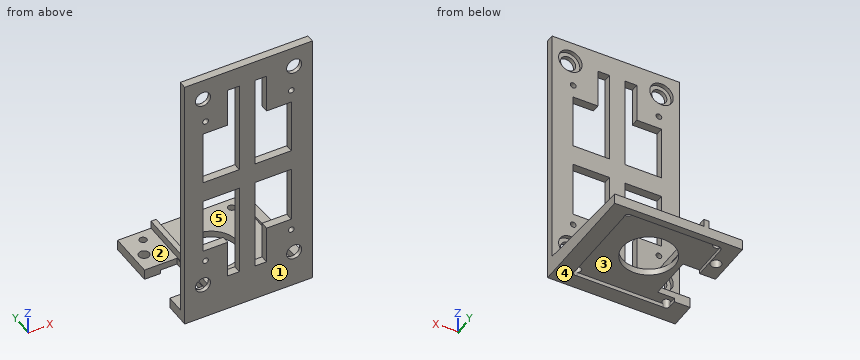
from build123d import *

# Parameters (mm, degrees)
SKETCH_1_R           = 2.9
SKETCH_1_R_2         = 1.1
EXTRUDE_1_DEPTH      = 3
SKETCH_2_R           = 4.5
CUT_EXTRUDE_1_DEPTH  = 1.5
SKETCH_3_W           = 49
SKETCH_3_H           = 4
EXTRUDE_2_DEPTH      = 42
EXTRUDE_2_DEPTH_BACK = 3
SKETCH_4_R           = 1.4
SKETCH_4_W           = 14.760499622
SKETCH_4_H           = 17
SKETCH_4_R_2         = 10
SKETCH_4_R_3         = 2
CUT_EXTRUDE_2_DEPTH  = 5
SKETCH_5_R           = 10
CUT_EXTRUDE_3_DEPTH  = 1.5
EXTRUDE_4_DEPTH      = 3.5
SKETCH_9_W           = 2
SKETCH_9_H           = 3
EXTRUDE_5_DEPTH      = 42
SKETCH_10_W          = 3
SKETCH_10_H          = 5.066593596
EXTRUDE_6_DEPTH      = 21


with BuildPart() as part:
    # 草图1 → 凸台-拉伸1 (new body)
    with BuildSketch(Plane(origin=(0, 0, 0), x_dir=(1, 0, 0), z_dir=(0, 1, 0))):
        Polygon((-42, 46), (-42, -1), (-42, -48), (0, -48), (7, -48), (7, 47), (7, 50), (-42, 50), align=None)
        with Locations((-35, -40)):
            Circle(SKETCH_1_R, mode=Mode.SUBTRACT)
        with Locations((-34, -30)):
            Circle(SKETCH_1_R_2, mode=Mode.SUBTRACT)
        Polygon((-35, -25), (-35, -4), (-21.05, -4), (-21.05, -40), (-25.5, -40), (-25.5, -25), align=None, mode=Mode.SUBTRACT)
        with Locations((0, -40)):
            Circle(SKETCH_1_R, mode=Mode.SUBTRACT)
        with Locations((-1.1, -30)):
            Circle(SKETCH_1_R_2, mode=Mode.SUBTRACT)
        Polygon((-1.1, -4), (-1.1, -25), (-10.6, -25), (-10.6, -40), (-15.05, -40), (-15.05, -4), align=None, mode=Mode.SUBTRACT)
        Polygon((-21.05, 4), (-35, 4), (-35, 25.5), (-25.5, 25.5), (-25.5, 40), (-21.05, 40), align=None, mode=Mode.SUBTRACT)
        with Locations((-34, 30)):
            Circle(SKETCH_1_R_2, mode=Mode.SUBTRACT)
        with Locations((-35, 40)):
            Circle(SKETCH_1_R, mode=Mode.SUBTRACT)
        Polygon((-10.6, 25.5), (-1.1, 25.5), (-1.1, 4), (-15.05, 4), (-15.05, 40), (-10.6, 40), align=None, mode=Mode.SUBTRACT)
        with Locations((-1.1, 30)):
            Circle(SKETCH_1_R_2, mode=Mode.SUBTRACT)
        with Locations((0, 40)):
            Circle(SKETCH_1_R, mode=Mode.SUBTRACT)
    extrude(amount=EXTRUDE_1_DEPTH)

    # 草图2 → 切除-拉伸1 (cut)
    with BuildSketch(Plane(origin=(0, 3, 0), x_dir=(1, 0, 0), z_dir=(0, 1, 0))):
        with Locations((-35, 40)):
            Circle(SKETCH_2_R)
        with Locations((0, 40)):
            Circle(SKETCH_2_R)
        with Locations((0, -40)):
            Circle(SKETCH_2_R)
        with Locations((-35, -40)):
            Circle(SKETCH_2_R)
    extrude(amount=-CUT_EXTRUDE_1_DEPTH, mode=Mode.SUBTRACT)

    # 草图3 → 凸台-拉伸2 (add, two sides)
    with BuildSketch(Plane(origin=(0, 3, 0), x_dir=(1, 0, 0), z_dir=(0, 1, 0))) as extrude_2_sk:
        with Locations((-17.5, 52)):
            Rectangle(SKETCH_3_W, SKETCH_3_H)
    extrude(amount=EXTRUDE_2_DEPTH)
    extrude(extrude_2_sk.sketch, amount=-EXTRUDE_2_DEPTH_BACK)

    # 草图4 → 切除-拉伸2 (cut, through all)
    with BuildSketch(Plane.XY.offset(-50)):
        with Locations((-34.5, 7)):
            Circle(SKETCH_4_R)
        with Locations((-36.880249811, 18.5)):
            Rectangle(SKETCH_4_W, SKETCH_4_H)
        with Locations((-34.5, 41)):
            Circle(SKETCH_4_R)
        with Locations((-0.5, 41)):
            Circle(SKETCH_4_R)
        with Locations((-0.5, 7)):
            Circle(SKETCH_4_R)
        with Locations((-17.5, 25)):
            Circle(SKETCH_4_R_2)
        with Locations((-38.080040601, 34.130797069)):
            Circle(SKETCH_4_R_3)
    extrude(amount=-CUT_EXTRUDE_2_DEPTH, mode=Mode.SUBTRACT)

    # 草图5 → 切除-拉伸3 (cut)
    with BuildSketch(Plane(origin=(0, 0, -54), x_dir=(-1, 0, 0), z_dir=(0, 0, -1))):
        with BuildLine():
            ThreePointArc((1.9, 41), (0.835827548, 39.640875334), (-0.738885511, 40.347954994))
            Line((-0.738885511, 40.347954994), (-0.738885511, 7.652045006))
            ThreePointArc((-0.738885511, 7.652045006), (0.835827548, 8.359124666), (1.9, 7))
            ThreePointArc((1.9, 7), (1.644381785, 6.193532189), (0.970870956, 5.681561324))
            Line((0.970870956, 5.681561324), (34.029129044, 5.681561324))
            ThreePointArc((34.029129044, 5.681561324), (33.693532189, 8.144381785), (35.9, 7))
            Line((35.9, 7), (35.9, 10))
            Line((35.9, 10), (29.5, 10))
            Line((29.5, 10), (29.5, 27))
            Line((29.5, 27), (35.9, 27))
            Line((35.9, 27), (35.9, 41))
            ThreePointArc((35.9, 41), (33.616753245, 39.913779411), (34.214464044, 42.370572588))
            Line((34.214464044, 42.370572588), (0.785535956, 42.370572588))
            ThreePointArc((0.785535956, 42.370572588), (1.586220589, 41.883246755), (1.9, 41))
        make_face()
        with Locations((17.5, 25)):
            Circle(SKETCH_5_R, mode=Mode.SUBTRACT)
    extrude(amount=-CUT_EXTRUDE_3_DEPTH, mode=Mode.SUBTRACT)

    # 草图7 → 凸台-拉伸4 (add)
    with BuildSketch(Plane(origin=(7, 0, 0), x_dir=(0, 0, -1), z_dir=(1, 0, 0))):
        Polygon((50, 3), (47, 3), (50, 45), align=None)
    extrude(amount=-EXTRUDE_4_DEPTH)

    # 草图9 → 凸台-拉伸5 (add)
    with BuildSketch(Plane(origin=(0, 3, 0), x_dir=(1, 0, 0), z_dir=(0, 1, 0))):
        with Locations((-28.188676473, 48.5)):
            Rectangle(SKETCH_9_W, SKETCH_9_H)
    extrude(amount=EXTRUDE_5_DEPTH)

    # 草图10 → 凸台-拉伸6 (add)
    with BuildSketch(Plane(origin=(-27.188676473, 0, 0), x_dir=(0, 0, -1), z_dir=(1, 0, 0))):
        with Locations((48.5, 5.533296798)):
            Rectangle(SKETCH_10_W, SKETCH_10_H)
    extrude(amount=EXTRUDE_6_DEPTH)


solid = part.part
Can you work these out from the model? Positions are in its coordinate system, mm. Face numbers are marked on the shaded views. A direction names the side the tool comes from. Coordinates: 2 decimals unless noted, no trailing zeros. Order: outer loops, then holes, each group sorted by start corner. A loop starts at its lowest first (then second) coordinate and runs counter-clockwise, first axis right, second up. Notation, with made-up numbers: (53.25, 82) -> (57.25, 82) arc R26 ccw to (57.25, 121) -> close; hole circle Ø5 at (28.5, -22). An arc over 180 degrees is marked (long way). Use one line per item in the form item = value.
Q1. Imagine slicing it at A-A, the plane z = 19.5. List the corners of the cut face in (x, y) for me, then the cut area to 3 significant figures.
From the geometry:
outline = (-42, 0) -> (-35, 0) -> (-35, 3) -> (-42, 3) -> close; (-21.05, 0) -> (-15.05, 0) -> (-15.05, 3) -> (-21.05, 3) -> close; (-1.1, 0) -> (7, 0) -> (7, 3) -> (-1.1, 3) -> close
area = 63.3 mm²
Q2. We'd pull the mould along X, two halves only. Please class the marked faces 3, 4 and 5: released by +X, released by -X, zero draft, split by the parting line, or undercut.
From the geometry:
face_3 = undercut
face_4 = zero draft
face_5 = undercut
Q3. Imagine slicing it at B-B, the plane x = -17.5. List the corners of the cut face in (y, z) for me.
From the geometry:
outline = (0, -54) -> (5.68, -54) -> (5.68, -52.5) -> (15, -52.5) -> (15, -50) -> (8.07, -50) -> (8.07, -47) -> (3, -47) -> (3, 48) -> (0, 48) -> close; (35, -52.5) -> (42.37, -52.5) -> (42.37, -54) -> (45, -54) -> (45, -50) -> (35, -50) -> close
Q4. Imagine slicing it at C-C, the plane y = 21. List the corners of the cut face in (x, z) for me, then the cut area to 3 significant figures.
From the geometry:
outline = (-29.5, -52.5) -> (-26.67, -52.5) -> (-26.67, -50) -> (-27.19, -50) -> (-27.19, -47) -> (-29.19, -47) -> (-29.19, -50) -> (-29.5, -50) -> close; (-8.33, -52.5) -> (0.74, -52.5) -> (0.74, -54) -> (7, -54) -> (7, -48.29) -> (3.5, -48.29) -> (3.5, -50) -> (-8.33, -50) -> close
area = 66.8 mm²
Q5. Will these pins go through, and if not, where does the flat tip stop? P1, Ø2, axis at x = -30, y = 18.5, coming from the +Z side; P2, Ø3.5, axis at x = -1.1, z = 30, coming from the +Y side; P3, Ø2, axis at x = -33.5, y = 30, coming from the -Z side.
From the geometry:
P1 = -47
P2 = 3
P3 = -52.5
Q6. I need wall thicknesses on L1, parallel to Y at x = -34.5, z = -52.4; L2, parallel to Y at x = -0.5, z = -51.85; L3, parallel to Y at x = 0, z = -51. Which ranges of each line are inside material? Lowest first, please.
From the geometry:
L1 = 0 to 5.6, 8.4 to 10, 27 to 39.6, 42.4 to 45
L2 = 0 to 5.6, 8.4 to 39.6, 42.4 to 45
L3 = 0 to 5.69, 8.31 to 39.69, 42.31 to 45
Q7. Which directions (+Z, -Z, +X, -X, +Y, -Y) give clear straight access to the entire face, cutting with the end or side of a thin tool? Please do the marked faces 1 and 2.
From the geometry:
face_1 = +Z, -Z, +X, -X, -Y
face_2 = +Z, -X, +Y
Q8. Imagine slicing it at D-D, the plane z = -30. List the corners of the cut face in (x, y) for me.
From the geometry:
outline = (-42, 0) -> (-35.1, 0) -> (-35.1, 3) -> (-42, 3) -> close; (-32.9, 0) -> (-25.5, 0) -> (-25.5, 3) -> (-32.9, 3) -> close; (-21.05, 0) -> (-15.05, 0) -> (-15.05, 3) -> (-21.05, 3) -> close; (-10.6, 0) -> (-2.2, 0) -> (-2.2, 3) -> (-10.6, 3) -> close; (0, 0) -> (7, 0) -> (7, 3) -> (0, 3) -> close
